Can you work these out from the model? Positions are in its coordinate system, mm. A direction names the side the tool comes from. Give positions to 0.01 mm unless a question says otherwise; leave off trailing zeros. Order: outer loops, then holes, each group sorted by start corner. A loop starts at its lowest first (then second) coordinate and runs counter-clockwise, first axis right, second up. Notation, with made-up numbers: (14.5, 73.5) - (38.5, 73.5) arc R9 cw to (38.5, 87.5) - close; hole circle Ø6 at (50, 74). An arc over 180 degrees is marked (long way). Use one line per item in the form item = value. Start each with the question number.
1) Suppose I cut it at D-D, the plane z = -2.5. Write out the boundary of the cut face in (x, y).
2) Which directions (+Z, -Z, +X, -X, +Y, -Y) give clear straight access to the entire face, cutting with the end or side of a thin tool? Please do faces 4 (the flat face through (-7, -370, 10.348)), 5 (the flat face through (-56.607, -370, 361)), 6 (the flat face through (794, -370, 110.348)), 7 (the flat face through (-7, -370, 410.348)), 8 (the flat face through (743.393, -370, 361)).
3) For pin 1 (12 mm diameter, centred on x = 304, z = 284.5, fed in from +Y); pin 2 (4 mm diameter, centred on x = 198, z = 30, fed in from -Y), each with a flat end and sliding along its axis, tell me the tip position at first contact or that it passes through.
4) Please list where these lines run through material, in increasing order: probe 1 along X at (y, z) = (-127, 27); probe 2 along Z at (x, y) = (793.5, -286.5); probe 3 along X at (y, z) = (-526, 376).
5) We'd pull the mould along Y, two halves only. Please class faces 1 (the flat face through (794, -725, 61)), 2 (the cylindrical face through (-3.353, -100.213, 361.048)), 3 (the flat face through (843.393, -370, 361)): released by +Y, released by -Y, zero draft, split by the parting line, or undercut.
6) Suppose I cut it at A-A, the plane y = -46.5. Write out the boundary of the cut face in (x, z), and give its area (3 significant figures).
7) Suppose I cut it at B-B, the plane y = -125. State how many separate pieces and enclosed holes the cut face has, and give its area (3 significant figures).
8) Suppose I cut it at C-C, the plane x = 441.5. Write out the boundary of the cut face in (y, z), and give its area (3 significant figures).
```python
from build123d import *

# Parameters (mm, degrees)
F0_W     = 500
F0_H     = 250
F1_DEPTH = 25
F2_W     = 100
F2_H     = 100
F3_DEPTH = 725
F5_D     = 50


with BuildPart() as f1:
    # F0 (on Front) → F1 (new body)
    with BuildSketch(Plane.XZ):
        with Locations((143.392576, 85.347861)):
            Rectangle(F0_W, F0_H)
    extrude(amount=F1_DEPTH)

    # F2 (on Front) → F3 (join)
    with BuildSketch(Plane.XZ):
        with Locations((-6.607424, 60.347861)):
            Rectangle(F2_W, F2_H)
    extrude(amount=F3_DEPTH)

    # F5 (through all)
    with Locations(Plane.XY.offset(110.347861)):
        with Locations((-6.607424, -125), (-6.607424, -325), (-6.607424, -525)):
            Hole(F5_D / 2)

    # F7: F1 across plane


with BuildPart() as f1_1:
    add(f1.part)
    add(f1.part.mirror(Plane(origin=(393.392576, -12.5, 85.347861), x_dir=(0, 1, 0), z_dir=(1, 0, 0))))

    # F9: F1 across plane


with BuildPart() as f1_2:
    add(f1_1.part)
    add(f1_1.part.mirror(Plane(origin=(393.392576, -12.5, 210.347861), x_dir=(1, 0, 0), z_dir=(0, 0, 1))))


solid = f1_2.part
```
Result sheet:
q1.outline = (-106.61, -25) - (893.39, -25) - (893.39, 0) - (-106.61, 0) - close
q2.face_4 = -Z, +X, -X, -Y
q2.face_5 = +Z, -Z, -X, -Y
q2.face_6 = +X, -X, -Y
q2.face_7 = +Z, +X, -X, -Y
q2.face_8 = +Z, -Z, -Y
q3.pin_1 = 0
q3.pin_2 = -25
q4.probe_1 = -56.61 to -31.53, 18.31 to 43.39, 743.39 to 768.47, 818.31 to 843.39
q4.probe_2 = 10.35 to 110.35, 310.35 to 410.35
q4.probe_3 = -56.61 to -31.59, 18.37 to 43.39, 743.39 to 768.41, 818.37 to 843.39
q5.face_1 = released by -Y
q5.face_2 = undercut
q5.face_3 = zero draft
q6.outline = (-56.61, 10.35) - (43.39, 10.35) - (43.39, 110.35) - (-56.61, 110.35) - close; (-56.61, 310.35) - (43.39, 310.35) - (43.39, 410.35) - (-56.61, 410.35) - close; (743.39, 10.35) - (843.39, 10.35) - (843.39, 110.35) - (743.39, 110.35) - close; (743.39, 310.35) - (843.39, 310.35) - (843.39, 410.35) - (743.39, 410.35) - close
q6.area = 40,000 mm²
q7.separate_pieces = 8
q7.enclosed_holes = 0
q7.area = 20,000 mm²
q8.outline = (-25, -39.65) - (0, -39.65) - (0, 460.35) - (-25, 460.35) - close
q8.area = 12,500 mm²
